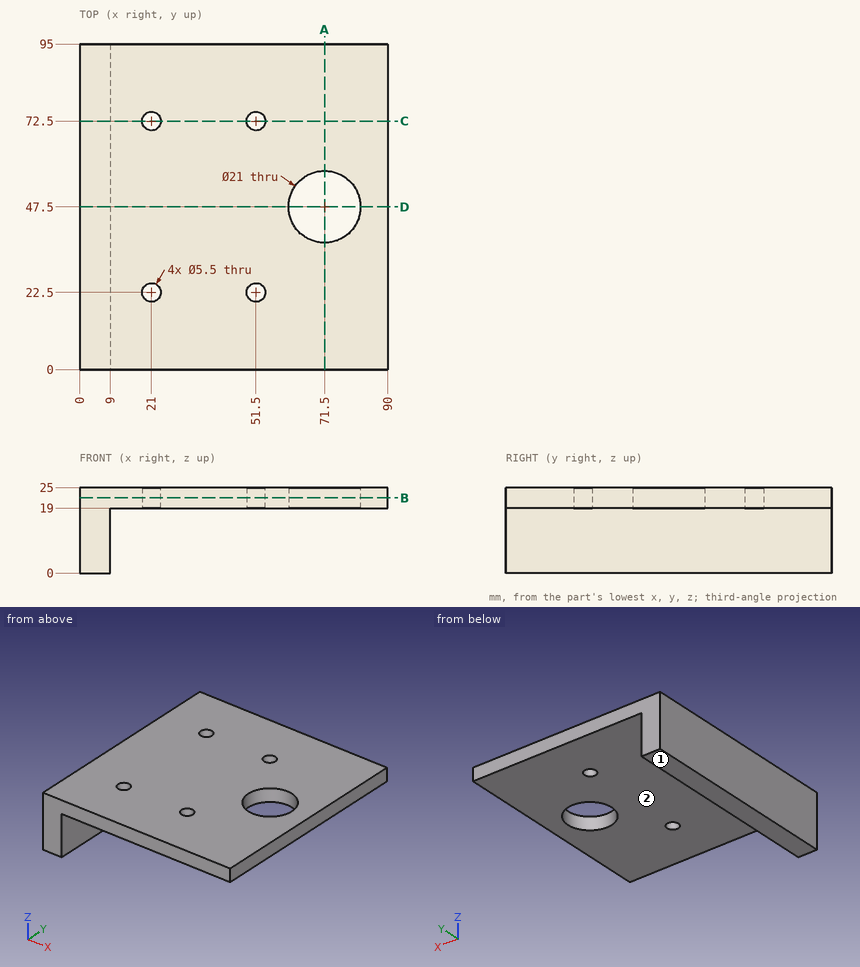
Source: three-view drawing plus pictorial views. Frame: mm from the lowest corner of the part. A direction names the side the tool comes from. Coordinates: 2 decimals unless noted, no trailing zeros. Order: outer loops, then holes, each group sorted by start corner. A loop starts at its lowest first (then second) coordinate and runs counter-clockwise, first axis right, second up.
Item 1: Cut plane A-A (x = 71.5). Return loops of the section in (y, z).
Output values:
outline: (0, 19) - (37, 19) - (37, 25) - (0, 25) - close; (58, 19) - (95, 19) - (95, 25) - (58, 25) - close
Item 2: Cut plane D-D (y = 47.5). Return loops of the section in (x, z), plus the area to 3 significant figures.
Output values:
outline: (0, 0) - (9, 0) - (9, 19) - (61, 19) - (61, 25) - (0, 25) - close; (82, 19) - (90, 19) - (90, 25) - (82, 25) - close
area: 585 mm2
Item 3: First-contact query: P1, Ø9, axis at x = 51.5, y = 72.5, coming from the -Z side; P2, Ø5, axis at y = 79, z = 6.5, coming from the +X side. Flat tips, straight axial feed; report the tip coordinate or a pass-through.
Output values:
P1: stops at z = 19
P2: stops at x = 9
Item 4: Material intervals for line 1 (X direction, y = 22.5, z = 20.5); line 2 (Y direction, x = 21, z = 22); line 3 (Z direction, x = 84, y = 55), sorted ascending.
Output values:
line 1: x = 0 to 18.25, 23.75 to 48.75, 54.25 to 90
line 2: y = 0 to 19.75, 25.25 to 69.75, 75.25 to 95
line 3: z = 19 to 25
Item 5: Set-up query: the marked faces 1 and 2. Return all of +Z, -Z, +X, -X, +Y, -Y with unobstructed straight access to the full face (end or side cutting, diameter ignored); none if empty.
Output values:
face 1: -Z, +X, -X, +Y, -Y
face 2: -Z, +X, +Y, -Y
Item 6: Cut plane B-B (z = 22). Return loops of the section in (x, y), plus the area to 3 significant figures.
Output values:
outline: (0, 0) - (90, 0) - (90, 95) - (0, 95) - close; hole circle Ø5.5 at (21, 22.5); hole circle Ø5.5 at (21, 72.5); hole circle Ø5.5 at (51.5, 22.5); hole circle Ø5.5 at (51.5, 72.5); hole circle Ø21 at (71.5, 47.5)
area: 8,110 mm2
Item 7: Cut plane C-C (y = 72.5). Return loops of the section in (x, z).
Output values:
outline: (0, 0) - (9, 0) - (9, 19) - (18.25, 19) - (18.25, 25) - (0, 25) - close; (23.75, 19) - (48.75, 19) - (48.75, 25) - (23.75, 25) - close; (54.25, 19) - (90, 19) - (90, 25) - (54.25, 25) - close
